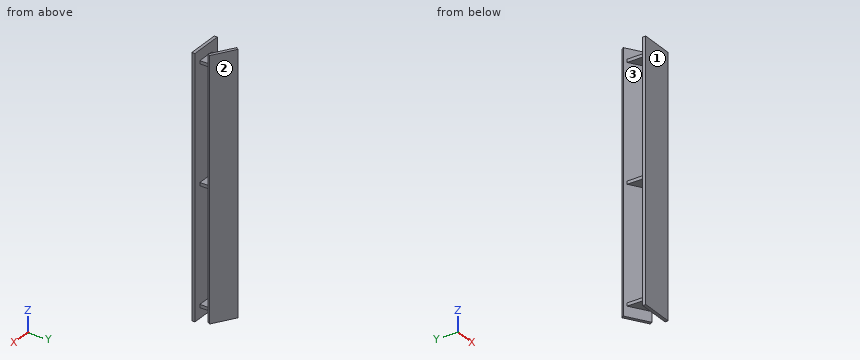
```python
from build123d import *

# Parameters (mm, degrees)
SKETCH_1_W                      = 64
SKETCH_1_H                      = 6
BASE_PLATE_940_TO_1004_T6_DEPTH = 500
INCLINED_BEARING_PLATE_T6_DEPTH = 500
TOE_WEB_1_T6_START              = 20
TOE_WEB_1_T6_DEPTH              = 6
TOE_WEB_2_T6_START              = 247
TOE_WEB_2_T6_DEPTH              = 6
TOE_WEB_3_T6_START              = 474
TOE_WEB_3_T6_DEPTH              = 6


with BuildPart() as part:
    # 草图1 → Base_plate_940_to_1004_t6 (new body)
    with BuildSketch(Plane.XY):
        with Locations((972, 3)):
            Rectangle(SKETCH_1_W, SKETCH_1_H)
    extrude(amount=BASE_PLATE_940_TO_1004_T6_DEPTH)



with BuildPart() as body_2:
    # 草图2 → Inclined_bearing_plate_t6 (new body)
    with BuildSketch(Plane.XY):
        Polygon((953.526014292, 55.936634693), (995.928419099, 29.440671481), (992.748903514, 24.352382904), (950.346498706, 50.848346116), align=None)
    extrude(amount=INCLINED_BEARING_PLATE_T6_DEPTH)


with BuildPart() as part_1:
    add(part.part)

    add(body_2.part)  # Toe_web_1_t6 merges body 2
    # 草图3 → Toe_web_1_t6 (add)
    with BuildSketch(Plane.XY.offset(TOE_WEB_1_T6_START)):
        Polygon((956, 6), (990, 6), (990, 26.070088461), (956, 47.315646426), align=None)
    extrude(amount=TOE_WEB_1_T6_DEPTH)

    # 草图4 → Toe_web_2_t6 (add)
    with BuildSketch(Plane.XY.offset(TOE_WEB_2_T6_START)):
        Polygon((956, 6), (990, 6), (990, 26.070088461), (956, 47.315646426), align=None)
    extrude(amount=TOE_WEB_2_T6_DEPTH)

    # 草图5 → Toe_web_3_t6 (add)
    with BuildSketch(Plane.XY.offset(TOE_WEB_3_T6_START)):
        Polygon((956, 6), (990, 6), (990, 26.070088461), (956, 47.315646426), align=None)
    extrude(amount=TOE_WEB_3_T6_DEPTH)


solid = part_1.part
```
The listing builds one solid part. Answer for the finished solid, in the listing's coordinates (mm). Face numbers are marked on the shaded views. Give positions to 0.01 mm unless a question says otherwise; leave off trailing zeros. Loops run counter-clockwise (first coordinate to the right, second up) from the corner with the lowest first, then second, coordinate; pieces in that order, holes last. Notation, with made-up numbers: M 35,69.25 L 44,69.25 A24 ccw 44,93.25 Z; hole C -9.5,-39 d7. An arc over 180 degrees is marked long. One line per item, written item: value.
1. Section A-A on z = 117.5 is taken. Determine the outline of the cut face in (x, y).
Found:
outline: M 940,0 L 1004,0 L 1004,6 L 940,6 Z; M 950.35,50.85 L 992.75,24.35 L 995.93,29.44 L 953.53,55.94 Z
2. For a pull along Y with two mould halves and no side action, classify the marked faces 1, 2 and 3 as pulls with the +Y half, pulls with the -Y half, needs draft (parallel to the pull), parting line crosses it, or undercut.
Found:
face 1: pulls with the -Y half
face 2: pulls with the +Y half
face 3: undercut
3. Section C-C on x = 970 is taken. Determine the outline of the cut face in (y, z), plus the area to 3 significant figures.
Found:
outline: M 0,0 L 6,0 L 6,20 L 38.57,20 L 38.57,0 L 45.64,0 L 45.64,500 L 38.57,500 L 38.57,480 L 6,480 L 6,500 L 0,500 Z; hole M 6,26 L 38.57,26 L 38.57,247 L 6,247 Z; hole M 6,253 L 38.57,253 L 38.57,474 L 6,474 Z
area: 7,120 mm^2
4. Section D-D on y = 37 is taken. Determine the outline of the cut face in (x, z).
Found:
outline: M 956,20 L 972.51,20 L 972.51,0 L 983.83,0 L 983.83,500 L 972.51,500 L 972.51,480 L 956,480 L 956,474 L 972.51,474 L 972.51,253 L 956,253 L 956,247 L 972.51,247 L 972.51,26 L 956,26 Z
5. Find the intervals of material crossed by probe 1 along Z at (x, y) = (970.5, 24.5); probe 2 along Y at (x, z) = (996.5, 417); probe 3 along Y at (x, z) = (974, 303), in increasing order.
Found:
probe 1: 20 to 26, 247 to 253, 474 to 480
probe 2: 0 to 6
probe 3: 0 to 6, 36.07 to 43.14
6. Each of these flat-tipped pins is pushed along its axis until it touches: P1, Ø1.8, axis at y = 23, z = 477, coming from the -X side; P2, Ø5, axis at x = 984.5, z = 157, coming from the +Y side; P3, Ø2, axis at y = 32.5, z = 382, coming from the -X side; P4, Ø10, axis at x = 984.5, z = 428, coming from the -Y side. Where does it stop, or does it pass through?
Found:
P1: x = 956
P2: y = 38.14
P3: x = 978.11
P4: y = 0
7. Section B-B on y = 12.5 is taken. Determine the outline of the cut face in (x, z).
Found:
outline: M 956,20 L 990,20 L 990,26 L 956,26 Z; M 956,247 L 990,247 L 990,253 L 956,253 Z; M 956,474 L 990,474 L 990,480 L 956,480 Z
